Drawing for the job (mm, zero at the part's lowest x, y, z). A direction names the side the tool comes from. Coordinates: 2 decimals unless noted, no trailing zeros. Loops run counter-clockwise (first coordinate to the right, second up) from the corner with the lowest first, then second, coordinate; pieces in that order, holes last. Notation, with made-up numbers: (-31, -38) - (21, -38) arc R25 ccw to (21, -6) - close; hole circle Ø10 at (-35.75, 1). An arc over 180 degrees is marked (long way). One line per item, written item: value.
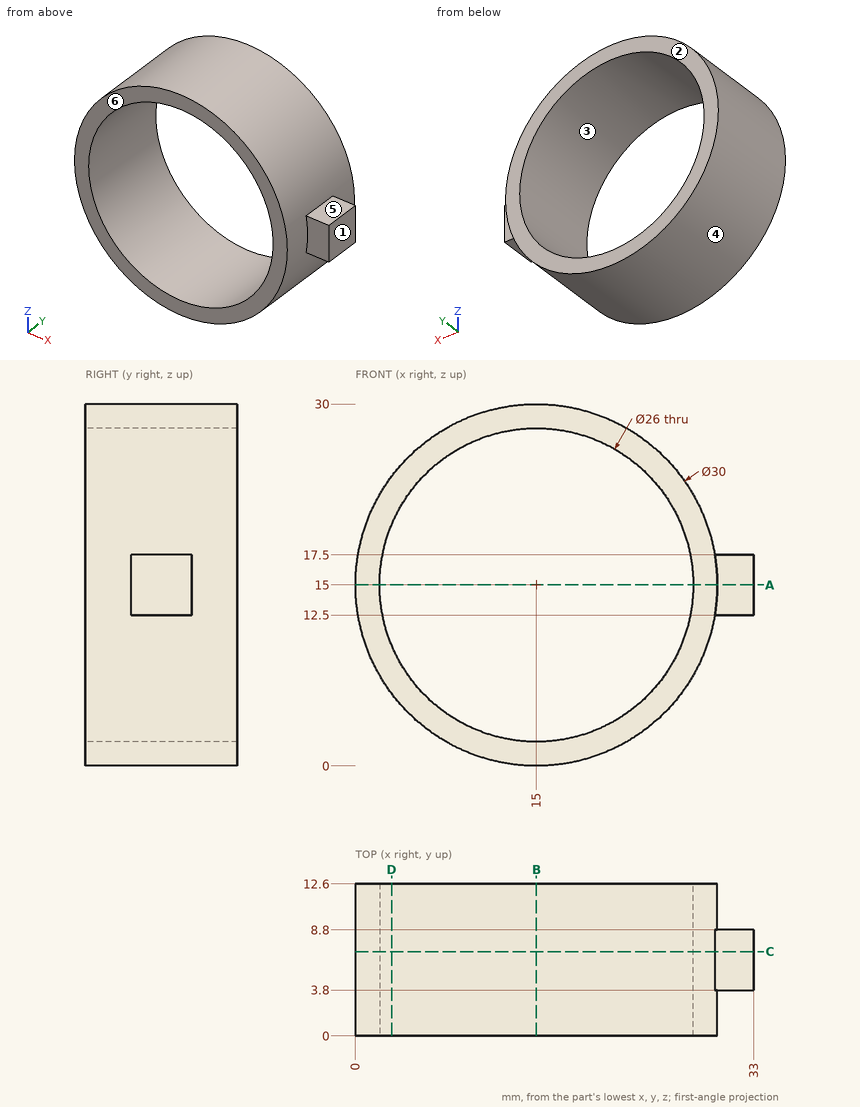
Item 1: Drop flat-ended pins along their axis: P1, Ø6, axis at y = 10.5, z = 22, coming from the +X side; P2, Ø4, axis at x = 17.5, z = 5, coming from the +Y side; P3, Ø1.5, axis at x = 16.5, y = 6, coming from the -Z side; P4, Ø1, axis at x = 31, z = 15.5, coming from the -Y side. Give the stop position or say it passes through.
Check result:
P1: stops at x = 29.46
P2: passes through
P3: stops at z = 0.02
P4: stops at y = 3.8
Item 2: Pull direction X, two halves, no side cores. Call the marked faces 1, 2, 3 and 4: released by +X, released by -X, zero draft, split by the parting line, or undercut.
Check result:
face 1: released by +X
face 2: zero draft
face 3: undercut
face 4: split by the parting line
Item 3: Cut at A-A, the plane z = 15. Write the cut outline in (x, y), then the cut area to 3 significant figures.
Check result:
outline: (0, 0) - (2, 0) - (2, 12.6) - (0, 12.6) - close; (28, 0) - (30, 0) - (30, 3.8) - (33, 3.8) - (33, 8.8) - (30, 8.8) - (30, 12.6) - (28, 12.6) - close
area: 65.4 mm^2
Item 4: Tool access for the marked faces 5 and 6: list every direction of +Z, -Z, +X, -X, +Y, -Y with a clear straight run to the whole face (end or side of a thin tool).
Check result:
face 5: +Z, +X, +Y, -Y
face 6: +Z, -Z, +X, -X, -Y
Item 5: Cut at D-D, the plane x = 3. Write the cut outline in (y, z).
Check result:
outline: (0, 6) - (12.6, 6) - (12.6, 10) - (0, 10) - close; (0, 20) - (12.6, 20) - (12.6, 24) - (0, 24) - close
Item 6: Probe probe 1 along Z at (x, y) = (15, 3.25); probe 2 along X at (y, z) = (8, 15). List the from-to ranges inside material, lowest first. Write a range as from..to.
Check result:
probe 1: z = 0..2, 28..30
probe 2: x = 0..2, 28..33
Item 7: Cut at C-C, the plane y = 7. Write the cut outline in (x, z), then the cut area to 3 significant figures.
Check result:
outline: (29.79, 12.5) - (33, 12.5) - (33, 17.5) - (29.79, 17.5) arc R15 ccw (long way) to start; hole circle Ø26 at (15, 15)
area: 191 mm^2
Item 8: Cut at B-B, the plane x = 15. Write the cut outline in (y, z).
Check result:
outline: (0, 0) - (12.6, 0) - (12.6, 2) - (0, 2) - close; (0, 28) - (12.6, 28) - (12.6, 30) - (0, 30) - close
